```python
from build123d import *

# Parameters (mm, degrees)
BOSS_EXTRUDE1_DEPTH     = 20.15
CUT_EXTRUDE1_DEPTH      = 40.134529676
CUT_EXTRUDE1_DEPTH_BACK = 40.134529676
CUT_EXTRUDE2_START      = -40.3
CUT_EXTRUDE2_DEPTH      = 3.9
SKETCH5_R               = 2.3
CUT_EXTRUDE3_DEPTH      = 39.164268799
SKETCH6_R               = 3.1
CUT_EXTRUDE4_DEPTH      = 39.164268799
SKETCH7_W               = 11.8
SKETCH7_H               = 4.7
SKETCH7_R               = 1
BOSS_EXTRUDE2_DEPTH     = 5
SKETCH8_W               = 4
SKETCH8_H               = 12
BOSS_EXTRUDE3_DEPTH     = 9.9
SKETCH8_2_W             = 4
SKETCH8_2_H             = 12
BOSS_EXTRUDE4_DEPTH     = 9.9
SKETCH9_W               = 11.8
SKETCH9_H               = 12
BOSS_EXTRUDE5_DEPTH     = 4
SKETCH10_R              = 3.1
BOSS_EXTRUDE6_DEPTH     = 2.2


with BuildPart() as part:
    # Sketch1 → Boss-Extrude1 (new, symmetric)
    with BuildSketch(Plane.XY):
        with BuildLine():
            Line((-27.023255814, 5), (27.023255814, 5))
            ThreePointArc((27.023255814, 5), (32.023255814, 0), (27.023255814, -5))
            Line((27.023255814, -5), (-27.023255814, -5))
            ThreePointArc((-27.023255814, -5), (-32.023255814, 0), (-27.023255814, 5))
        make_face()
    extrude(amount=BOSS_EXTRUDE1_DEPTH, both=True)

    # Sketch2 → Cut-Extrude1 (cut, two sides: drawn at the far end of the back side and taken through both)
    with BuildSketch(Plane(origin=(0, 5, 0), x_dir=(1, 0, 0), z_dir=(0, 1, 0)).offset(-CUT_EXTRUDE1_DEPTH_BACK)):
        Polygon((-2, -20.15), (-2, 20.15), (-27.023255814, 20.15), (-37.952019542, 20.15), (-37.952019542, -20.15), (-27.023255814, -20.15), align=None)
        Polygon((27.023255814, 15.35), (38.05829872, 15.35), (38.05829872, -15.35), (27.023255814, -15.35), (2, -15.35), (2, 15.35), align=None)
    extrude(amount=CUT_EXTRUDE1_DEPTH + CUT_EXTRUDE1_DEPTH_BACK, mode=Mode.SUBTRACT)

    # Sketch4 → Cut-Extrude2 (cut)
    with BuildSketch(Plane.XY.offset(20.15).offset(CUT_EXTRUDE2_START)):
        with BuildLine():
            Line((25.123749299, 2.85), (12.848255814, 1.9))
            ThreePointArc((12.848255814, 1.9), (10.948255814, 0), (12.848255814, -1.9))
            Line((12.848255814, -1.9), (25.123749299, -2.85))
            ThreePointArc((25.123749299, -2.85), (30.448255814, 0), (25.123749299, 2.85))
        make_face()
    extrude(amount=CUT_EXTRUDE2_DEPTH, mode=Mode.SUBTRACT)

    # Sketch5 → Cut-Extrude3 (cut, through all)
    with BuildSketch(Plane.XY):
        with Locations((27.023255814, 0)):
            Circle(SKETCH5_R)
    extrude(amount=-CUT_EXTRUDE3_DEPTH, mode=Mode.SUBTRACT)

    # Sketch6 → Cut-Extrude4 (cut, through all)
    with BuildSketch(Plane.XY):
        with Locations((27.023255814, 0)):
            Circle(SKETCH6_R)
    extrude(amount=CUT_EXTRUDE4_DEPTH, mode=Mode.SUBTRACT)

    # Sketch7 → Boss-Extrude2 (add)
    # profile 1 of 2: a face of its own
    with BuildSketch(Plane(origin=(0, 0, 0), x_dir=(1, 0, 0), z_dir=(0, 1, 0))):
        with Locations((-7.9, 13.6)):
            Rectangle(SKETCH7_W, SKETCH7_H)
        with Locations(Location((-7.9, 13.55, 0), (0, 0, 270))):
            Circle(SKETCH7_R, mode=Mode.SUBTRACT)
    # profile 2 of 2: a face of its own
    with BuildSketch(Plane(origin=(0, 0, 0), x_dir=(1, 0, 0), z_dir=(0, 1, 0))):
        with Locations((-7.9, -13.6)):
            Rectangle(SKETCH7_W, SKETCH7_H)
        with Locations(Location((-7.9, -13.65, 0), (0, 0, 270))):
            Circle(SKETCH7_R, mode=Mode.SUBTRACT)
    extrude(amount=-BOSS_EXTRUDE2_DEPTH)

    # Sketch8 → Boss-Extrude3 (add)
    with BuildSketch(Plane(origin=(0, 5, 0), x_dir=(1, 0, 0), z_dir=(0, 1, 0))):
        with Locations((0, 5.25)):
            Rectangle(SKETCH8_W, SKETCH8_H)
    extrude(amount=BOSS_EXTRUDE3_DEPTH)

    # Sketch8<2> → Boss-Extrude4 (add)
    with BuildSketch(Plane(origin=(0, 5, 0), x_dir=(1, 0, 0), z_dir=(0, 1, 0))):
        with Locations((0, 5.25)):
            Rectangle(SKETCH8_2_W, SKETCH8_2_H)
    extrude(amount=BOSS_EXTRUDE4_DEPTH)

    # Sketch9 → Boss-Extrude5 (add)
    with BuildSketch(Plane(origin=(0, 14.9, 0), x_dir=(1, 0, 0), z_dir=(0, 1, 0))):
        with Locations((-7.9, 5.25)):
            Rectangle(SKETCH9_W, SKETCH9_H)
    extrude(amount=-BOSS_EXTRUDE5_DEPTH)

    # Sketch10 → Boss-Extrude6 (add)
    with BuildSketch(Plane(origin=(0, 14.9, 0), x_dir=(1, 0, 0), z_dir=(0, 1, 0))):
        with Locations(Location((-7.9, 5.15, 0), (0, 0, 270))):
            Circle(SKETCH10_R)
    extrude(amount=BOSS_EXTRUDE6_DEPTH)


solid = part.part
```
Work out the finished part from the listing and answer in its coordinate system (mm). A direction names the side the tool comes from. Give positions to 0.01 mm unless a question says otherwise; leave off trailing zeros. Order: outer loops, then holes, each group sorted by start corner. A loop starts at its lowest first (then second) coordinate and runs counter-clockwise, first axis right, second up.
1. Section B-B, the plane z = -17 is taken. Determine the outline of the cut face in (x, y) (3 decimals).
Result sheet:
outline: (-2, -5) - (27.023, -5) arc R5 ccw to (27.023, 5) - (-2, 5) - close; hole (12.848, -1.9) - (25.124, -2.85) arc R3.425 ccw (long way) to (25.124, 2.85) - (12.848, 1.9) arc R1.9 ccw to start
2. The mould has two halves that part along Z. Classify faces 1 (the flat face through (2, 3, 0)), 2 (the flat face through (17, 0, 15.35)), 3 (the flat face through (-8, -2, -15.95)), 4 (the flat face through (-8, 0, 12.5)): released by +Z, released by -Z, zero draft, split by the parting line, or undercut.
Result sheet:
face 1: undercut
face 2: undercut
face 3: released by -Z
face 4: zero draft
3. Section D-D, the plane y = 1 is taken. Determine the outline of the cut face in (x, z), and give its area (3 significant figures).
Result sheet:
outline: (-2, -20.15) - (11.23, -20.15) - (11.23, -16.25) - (24.95, -16.25) - (24.95, -15.35) - (2, -15.35) - (2, 15.35) - (24.09, 15.35) - (24.09, 20.15) - (-2, 20.15) - close; (29.09, -16.25) - (30.3, -16.25) - (30.3, -20.15) - (31.92, -20.15) - (31.92, -15.35) - (29.09, -15.35) - close; (29.96, 15.35) - (31.92, 15.35) - (31.92, 20.15) - (29.96, 20.15) - close
area: 342 mm2
4. Straight lines are drawn through the part: L1, parallel to X at y = -3.6, z = -13.55; L2, parallel to X at y = 0, z = -17.6; L3, parallel to Z at x = 20, y = -0.5. For each, find the intervals that lie inside material, in ascending order.
Result sheet:
L1: x = -13.8 to -8.9, -6.9 to 2
L2: x = -2 to 10.95, 30.45 to 32.02
L3: z = -16.25 to -15.35, 15.35 to 20.15
5. Each of these flat-tipped pins is pushed along its axis until it touches: P1, Ø4, axis at x = 26.5, z = 13.5, coming from the +Y side; P2, Ø7, axis at x = 27.02, y = 0, coming from the +Z side; P3, Ø8, axis at y = 2.5, z = 10.5, coming from the +X side; P4, Ø2.5, axis at x = -9.5, y = -3.5, coming from the -Z side. Where does it stop, or does it pass through?
Result sheet:
P1: stops at y = 5
P2: stops at z = 20.15
P3: stops at x = 2
P4: stops at z = -15.95
6. Section C-C, the plane x = 9 is taken. Determine the outline of the cut face in (y, z).
Result sheet:
outline: (-5, -20.15) - (5, -20.15) - (5, -15.35) - (-5, -15.35) - close; (-5, 15.35) - (5, 15.35) - (5, 20.15) - (-5, 20.15) - close
7. Section A-A, the plane x = -7.9 is taken. Determine the outline of the cut face in (y, z).
Result sheet:
outline: (-5, -15.95) - (0, -15.95) - (0, -14.55) - (-5, -14.55) - close; (-5, -12.55) - (0, -12.55) - (0, -11.25) - (-5, -11.25) - close; (-5, 11.25) - (0, 11.25) - (0, 12.65) - (-5, 12.65) - close; (-5, 14.65) - (0, 14.65) - (0, 15.95) - (-5, 15.95) - close; (10.9, -11.25) - (14.9, -11.25) - (14.9, -8.25) - (17.1, -8.25) - (17.1, -2.05) - (14.9, -2.05) - (14.9, 0.75) - (10.9, 0.75) - close
8. For faces 5 (the flat face through (9, 5, 16)), 6 (the flat face through (-4, 12, -11.25)), 7 (the cylindrical face through (29.98, 0.93, 17.72)), 8 (the cylindrical face through (-10.926, 15.985, -5.822)), 9 (the flat face through (-8, 10.9, -5)), determine the directions among +Z, -Z, +X, -X, +Y, -Y from which every point of the face is accessible in a straight line to the end or side of a thin tool.
Result sheet:
face 5: +Z, +X, -X, +Y
face 6: -Z, +X, -X, +Y
face 7: +Z
face 8: +Y
face 9: +Z, -Z, -X, -Y
